Part model, mm, in its own coordinate system. Give positions to 0.01 mm unless a question says otherwise; leave off trailing zeros. Order: outer loops, then holes, each group sorted by start corner. A loop starts at its lowest first (then second) coordinate and runs counter-clockwise, first axis right, second up. Notation, with made-up numbers: (73, 74) - (116, 74) arc R17 cw to (116, 100) - close; hole circle Ø8 at (-2.75, -2). An arc over 180 degrees is marked (long way). One line per item, written item: value.
```python
from build123d import *

# Parameters (mm, degrees)
F0_W     = 50
F0_H     = 40
F1_DEPTH = 50
F2_R     = 10
F3_DEPTH = 25
F4_SIZE  = 5


with BuildPart() as f1:
    # F0 (on Front) → F1 (new body)
    with BuildSketch(Plane.XZ):
        with Locations((-9.473613, 1.82123)):
            Rectangle(F0_W, F0_H)
    extrude(amount=F1_DEPTH)

    # F2 (on face) → F3 (cut)
    with BuildSketch(Plane.XY.offset(21.82123)):
        with Locations((-14.10244, -27.554378)):
            Circle(F2_R)
    extrude(amount=-F3_DEPTH, mode=Mode.SUBTRACT)

    # F4
    f4_edges = [f1.edges().sort_by_distance(p)[0] for p in [
        (15.526387, -25, -18.17877),
    ]]
    chamfer(f4_edges, length=F4_SIZE)


solid = f1.part
```
1) Cut at D-D, the plane x = -21. Give the cut face in (y, z).
Outcome:
outline: (-50, -18.18) - (0, -18.18) - (0, 21.82) - (-20.31, 21.82) - (-20.31, -3.18) - (-34.79, -3.18) - (-34.79, 21.82) - (-50, 21.82) - close
2) Drill centre lines: line 1 along Y through (x, z) = (-14, 2); line 2 along Y through (x, z) = (-17, 10.5); line 3 along X through (y, z) = (-29.5, 13). Where is each one in solid material? Low to high. Write a range as from..to.
Outcome:
line 1: y = -50..-37.55, -17.55..0
line 2: y = -50..-37.13, -17.98..0
line 3: x = -34.47..-23.91, -4.29..15.53
3) Cut at B-B, the plane y = -35. Give the cut face in (x, z), then the cut area to 3 significant figures.
Outcome:
outline: (-34.47, -18.18) - (10.53, -18.18) - (15.53, -13.18) - (15.53, 21.82) - (-7.43, 21.82) - (-7.43, -3.18) - (-20.78, -3.18) - (-20.78, 21.82) - (-34.47, 21.82) - close
area: 1,650 mm^2
4) Cut at A-A, the plane x = -11. Give the cut face in (y, z).
Outcome:
outline: (-50, -18.18) - (0, -18.18) - (0, 21.82) - (-18.05, 21.82) - (-18.05, -3.18) - (-37.06, -3.18) - (-37.06, 21.82) - (-50, 21.82) - close
5) Mould opens along Y. For faces 1 (the flat face through (-4, -25, 21.821)), 2 (the flat face through (-10, 0, 2)), 3 (the cylindrical face through (-4.865, -31.384, 9.496)), 4 (the flat face through (-14, -27, -3.179)) say: released by +Y, released by -Y, zero draft, split by the parting line, or undercut.
Outcome:
face 1: zero draft
face 2: released by +Y
face 3: undercut
face 4: undercut
6) Cut at C-C, the plane z = 1. Give the cut face in (x, y).
Outcome:
outline: (-34.47, -50) - (15.53, -50) - (15.53, 0) - (-34.47, 0) - close; hole circle Ø20 at (-14.1, -27.55)
7) Pin check, flat tip, straight feed: pin 1 (2 mm diameter, centred on x = -6, y = -29.5, fed in from +Z). Stop position of the tip, or through.
Outcome:
pin 1: stops at z = -3.18
